```python
from build123d import *

# Parameters (mm, degrees)
BOSS_EXTRUDE3_DEPTH = 31
SKETCH3_R           = 1.65
SKETCH3_R_2         = 11
BOSS_EXTRUDE4_DEPTH = 6
SKETCH4_R           = 4
CUT_EXTRUDE1_DEPTH  = 6
SKETCH7_R           = 4
CUT_EXTRUDE2_DEPTH  = 75.371903297
SKETCH10_W          = 21.3
SKETCH10_H          = 6
BOSS_EXTRUDE6_DEPTH = 6
SKETCH11_W          = 25
SKETCH11_H          = 6
BOSS_EXTRUDE7_DEPTH = 5
BOSS_EXTRUDE8_DEPTH = 1


with BuildPart() as part:
    # Sketch2 → Boss-Extrude3 (new body)
    with BuildSketch(Plane(origin=(0, 0, 0), x_dir=(0, 1, 0), z_dir=(0, 0, 1))):
        Polygon((26, 0), (20, 0), (20, -20), (0, -20), (0, -26), (26, -26), align=None)
    extrude(amount=BOSS_EXTRUDE3_DEPTH)

    # Sketch3 → Boss-Extrude4 (add)
    with BuildSketch(Plane(origin=(0, 0, 0), x_dir=(1, 0, 0), z_dir=(0, 0, -1))):
        Polygon((68.3, -5), (26, -5), (26, -26), (26, -47.3), (68.3, -47.3), align=None)
        with Locations(Location((31.65, -41.65, 0), (0, 0, 180))):
            Circle(SKETCH3_R, mode=Mode.SUBTRACT)
        with Locations(Location((62.65, -41.65, 0), (0, 0, 180))):
            Circle(SKETCH3_R, mode=Mode.SUBTRACT)
        with Locations(Location((31.65, -10.65, 0), (0, 0, 180))):
            Circle(SKETCH3_R, mode=Mode.SUBTRACT)
        with Locations(Location((47.15, -26.15, 0), (0, 0, 180))):
            Circle(SKETCH3_R_2, mode=Mode.SUBTRACT)
        with Locations(Location((62.65, -10.65, 0), (0, 0, 180))):
            Circle(SKETCH3_R, mode=Mode.SUBTRACT)
    extrude(amount=-BOSS_EXTRUDE4_DEPTH)

    # Sketch4 → Cut-Extrude1 (cut)
    with BuildSketch(Plane.XZ.offset(-20)):
        with Locations((10, 7.5)):
            Circle(SKETCH4_R)
        with Locations((10, 23.5)):
            Circle(SKETCH4_R)
    extrude(amount=-CUT_EXTRUDE1_DEPTH, mode=Mode.SUBTRACT)

    # Sketch7 → Cut-Extrude2 (cut, through all)
    with BuildSketch(Plane(origin=(20, 0, 0), x_dir=(0, -1, 0), z_dir=(-1, 0, 0))):
        with Locations(Location((-10, 20.5, 0), (0, 0, 90))):
            Circle(SKETCH7_R)
        with Locations(Location((-10, 10.5, 0), (0, 0, 90))):
            Circle(SKETCH7_R)
    extrude(amount=-CUT_EXTRUDE2_DEPTH, mode=Mode.SUBTRACT)

    # Sketch10 → Boss-Extrude6 (add)
    with BuildSketch(Plane(origin=(26, 0, 0), x_dir=(0, -1, 0), z_dir=(-1, 0, 0))):
        with Locations((-36.65, 3)):
            Rectangle(SKETCH10_W, SKETCH10_H)
        Polygon((-47.3, 6), (-26, 6), (-26, 22.3), (-31, 22.3), align=None)
    extrude(amount=BOSS_EXTRUDE6_DEPTH)

    # Sketch11 → Boss-Extrude7 (add)
    with BuildSketch(Plane.XZ.offset(-5)):
        Polygon((26, 31), (26, 6), (51, 6), align=None)
        with Locations((38.5, 3)):
            Rectangle(SKETCH11_W, SKETCH11_H)
    extrude(amount=BOSS_EXTRUDE7_DEPTH)

    # Sketch13 → Boss-Extrude8 (add)
    with BuildSketch(Plane(origin=(0, 5, 0), x_dir=(-1, 0, 0), z_dir=(0, 1, 0))):
        Polygon((-51, 6), (-26, 31), (-26, 6), align=None)
    extrude(amount=BOSS_EXTRUDE8_DEPTH)


solid = part.part
```
CAD build for the part. Positions are in the model's coordinates, mm. A direction names the side the tool comes from. Coordinates: 2 decimals unless noted, no trailing zeros. Write each loop counter-clockwise with the first axis right and the second up, starting at its lowest first coordinate (ties: lowest second). Pieces come first, ordered by that corner, then holes.
(1) 3-axis set-ups, long thin cutter, end or side, ignore diameter. For faces 5 (the face through (20, 10, 15)), 6 (the face through (23, 28, 22.3)), 7 (the face through (61.76, 43.04, 2.96)), 8 (the face through (56, 35, 6)), 9 (the face through (39, 3, 18)): which of +Z, -Z, +X, -X, +Y, -Y reach the whole face in a straight line?
(2) Flat gauge pins, fed straight in: pin 1 (6 mm diameter, centred on x = 28.5, z = 18, fed in from -Y); pin 2 (2 mm diameter, centred on x = 37, z = 12.5, fed in from +Y); pin 3 (3 mm diameter, centred on x = 55.5, y = 41, fed in from +Z); pin 4 (6.5 mm diameter, centred on y = 10, z = 10.5, fed in from -X). Where does each tip first touch, or does it go through?
(3) Cut at C-C, the plane x = 62.65. List the corners of the cut face in (y, z), and give its area (3 significant figures).
(4) Cut at A-A, the plane y = 24. List the corners of the cut face in (x, z).
(5) Drill centre lines: probe 1 along Y at (x, z) = (31.65, 1.65); probe 2 along X at (y, z) = (24.5, 5.5); probe 3 along Y at (x, z) = (31, 3). Where is each one in solid material? Low to high.
(6) Cut at D-D, the plane z = 23.5. List the corners of the cut face in (x, y).
(7) Two-plate mould, pull along Y, no slides. Class faces 1 (the face through (30.126, 10.018, 2.958)), 2 (the face through (22.958, 10.176, 16.504)), 3 (the face through (51, 3, 3)), 4 (the face through (60, 5, 3)): +Y half, -Y half, draft (parallel to the pull), parting line (faces both ways), or undercut.
(8) Cut at B-B, the plane x = 47.15. List the corners of the cut face in (y, z).
Geometry says:
1. face 5: +Z, -Z, -X, -Y
1. face 6: +Z, +X, -X, +Y
1. face 7: +Z, -Z
1. face 8: +Z, +X, +Y
1. face 9: +Z, +X, +Y, -Y
2. pin 1: stops at y = 0
2. pin 2: stops at y = 6
2. pin 3: stops at z = 6
2. pin 4: passes through
3. outline: (5, 0) - (9, 0) - (9, 6) - (5, 6) - close; (12.3, 0) - (40, 0) - (40, 6) - (12.3, 6) - close; (43.3, 0) - (47.3, 0) - (47.3, 6) - (43.3, 6) - close
3. area: 214 mm2
4. outline: (0, 0) - (36.36, 0) - (36.36, 6) - (26, 6) - (26, 31) - (0, 31) - close; (57.94, 0) - (68.3, 0) - (68.3, 6) - (57.94, 6) - close; hole circle Ø8 at (10, 7.5); hole circle Ø8 at (10, 23.5)
5. probe 1: y = 0 to 9, 12.3 to 40, 43.3 to 47.3
5. probe 2: x = 0 to 6.54, 13.46 to 36.27, 58.03 to 68.3
5. probe 3: y = 0 to 9.13, 12.17 to 40.13, 43.17 to 47.3
6. outline: (0, 20) - (6, 20) - (6, 26) - (0, 26) - close; (14, 20) - (20, 20) - (20, 12.65) - (26, 12.65) - (26, 26) - (14, 26) - close; (20, 0) - (33.5, 0) - (33.5, 6) - (26, 6) - (26, 7.35) - (20, 7.35) - close
7. face 1: undercut
7. face 2: undercut
7. face 3: draft
7. face 4: -Y half
8. outline: (0, 0) - (15.15, 0) - (15.15, 6) - (6, 6) - (6, 9.85) - (0, 9.85) - close; (37.15, 0) - (47.3, 0) - (47.3, 6) - (37.15, 6) - close
